from build123d import *

# Parameters (mm, degrees)
SKETCH1_W           = 39
SKETCH1_H           = 16
SKETCH1_R           = 1.5
BOSS_EXTRUDE1_DEPTH = 2
SKETCH3_W           = 25.4
SKETCH3_H           = 6.35
SKETCH3_R           = 1.5
BOSS_EXTRUDE2_DEPTH = 2.5
BOSS_EXTRUDE3_DEPTH = 6.35
SKETCH5_W           = 8
SKETCH5_H           = 15.6
BOSS_EXTRUDE4_DEPTH = 10


with BuildPart() as part:
    # Sketch1 → Boss-Extrude1 (new body)
    with BuildSketch(Plane(origin=(0, 0, 0), x_dir=(1, 0, 0), z_dir=(0, 1, 0))):
        Rectangle(SKETCH1_W, SKETCH1_H)
        with Locations(Location((-16.5, -5, 0), (0, 0, 270))):
            Circle(SKETCH1_R, mode=Mode.SUBTRACT)
        with Locations(Location((2.5, -5, 0), (0, 0, 270))):
            Circle(SKETCH1_R, mode=Mode.SUBTRACT)
    extrude(amount=BOSS_EXTRUDE1_DEPTH)

    # Sketch3 → Boss-Extrude2 (add)
    with BuildSketch(Plane(origin=(0, 2, 0), x_dir=(1, 0, 0), z_dir=(0, 1, 0))):
        with Locations((-7, -5)):
            Rectangle(SKETCH3_W, SKETCH3_H)
        with Locations(Location((-16.5, -5, 0), (0, 0, 270))):
            Circle(SKETCH3_R, mode=Mode.SUBTRACT)
        with Locations(Location((2.5, -5, 0), (0, 0, 270))):
            Circle(SKETCH3_R, mode=Mode.SUBTRACT)
    extrude(amount=BOSS_EXTRUDE2_DEPTH)

    # Sketch4 → Boss-Extrude3 (add)
    with BuildSketch(Plane.XY.offset(8.175)):
        with BuildLine():
            Line((-8.8, 13.7), (-13.5, 13.7))
            Line((-13.5, 13.7), (-13.5, 4.5))
            Line((-13.5, 4.5), (-6.999999998, 4.5))
            ThreePointArc((-6.999999998, 4.5), (-8.272792205, 5.027207793), (-8.8, 6.3))
            Line((-8.8, 6.3), (-8.8, 13.7))
        make_face()
        with BuildLine():
            ThreePointArc((-5.2, 6.3), (-5.727207793, 5.027207795), (-6.999999998, 4.5))
            Line((-6.999999998, 4.5), (-0.5, 4.5))
            Line((-0.5, 4.5), (-0.5, 13.7))
            Line((-0.5, 13.7), (-5.2, 13.7))
            Line((-5.2, 13.7), (-5.2, 6.3))
        make_face()
    extrude(amount=-BOSS_EXTRUDE3_DEPTH)

    # Sketch5 → Boss-Extrude4 (add)
    with BuildSketch(Plane(origin=(0, 2, 0), x_dir=(1, 0, 0), z_dir=(0, 1, 0))):
        with Locations((15.3, 0)):
            Rectangle(SKETCH5_W, SKETCH5_H)
    extrude(amount=BOSS_EXTRUDE4_DEPTH)


solid = part.part
Here's how the part is built. I have some questions about the finished solid (model axes, mm). A direction names the side the tool comes from. Round coordinates to 2 decimals unless told otherwise and drop trailing zeros. Write each loop counter-clockwise with the first axis right and the second up, starting at its lowest first coordinate (ties: lowest second). Pieces come first, ordered by that corner, then holes.
1. If we mould it in two halves opening along Z, with no side actions, what happens to faces 1 (the cylindrical face through (1.17, 2.22, 5.69)), 2 (the flat face through (0, 1, -8)), 3 (the flat face through (15, 12, 0)), 4 (the flat face through (-4, 7, 8.175))? For each: released by +Z, released by -Z, zero draft, split by the parting line, or undercut.
2. Suppose I cut it at B-B (x = -16.5). List the corners of the cut face in (y, z) for me (3 decimals), and give its area (3 significant figures).
3. Suppose I cut it at A-A (y = 8.25). List the corners of the cut face in (x, z) for me (3 decimals), and give its area (3 significant figures).
4. Suppose I cut it at C-C (z = 5). List the corners of the cut face in (x, y) for me.
5. Suppose I cut it at D-D (z = -4). List the corners of the cut face in (x, y) for me.
6. For faces 5 (the flat face through (-5.2, 10, 5)), 6 (the flat face through (15, 7, 7.8)), 7 (the flat face through (-4, 7, 1.825)), 8 (the flat face through (-13.5, 9, 5)), which set-ups out of +Z, -Z, +X, -X, +Y, -Y let a thin tool reach every point of the face, with its end or its side?
7. Will these pins go through, and if not, where does the flat tip stop? pin 1 Ø8 at (x, y) = (6.5, 11) entering from +Z; pin 2 Ø6 at (x, z) = (4, 0.5) entering from +Y; pin 3 Ø1.9 at (y, z) = (8, 4.5) entering from -X; pin 4 Ø8 at (x, z) = (-7, -3.5) entering from +Y.
8. I need wall thicknesses on L1, parallel to X at y = 7.5, z = 5; L2, parallel to X at y = 1.9, z = 5; L3, parallel to X at y = 2.8, z = 5. Which ranges of each line are inside material? Lowest first, please.
Answer sheet:
1. face 1: undercut
1. face 2: released by -Z
1. face 3: zero draft
1. face 4: released by +Z
2. outline: (0, -8) - (2, -8) - (2, 1.825) - (4.5, 1.825) - (4.5, 3.5) - (0, 3.5) - close; (0, 6.5) - (4.5, 6.5) - (4.5, 8.175) - (2, 8.175) - (2, 8) - (0, 8) - close
2. area: 34.4 mm2
3. outline: (-13.5, 1.825) - (-8.8, 1.825) - (-8.8, 8.175) - (-13.5, 8.175) - close; (-5.2, 1.825) - (-0.5, 1.825) - (-0.5, 8.175) - (-5.2, 8.175) - close; (11.3, -7.8) - (19.3, -7.8) - (19.3, 7.8) - (11.3, 7.8) - close
3. area: 184 mm2
4. outline: (-19.7, 2) - (-19.5, 2) - (-19.5, 0) - (-18, 0) - (-18, 4.5) - (-19.7, 4.5) - close; (-15, 0) - (1, 0) - (1, 4.5) - (-0.5, 4.5) - (-0.5, 13.7) - (-5.2, 13.7) - (-5.2, 6.3) arc R1.8 cw to (-8.8, 6.3) - (-8.8, 13.7) - (-13.5, 13.7) - (-13.5, 4.5) - (-15, 4.5) - close; (4, 0) - (19.5, 0) - (19.5, 2) - (19.3, 2) - (19.3, 12) - (11.3, 12) - (11.3, 2) - (5.7, 2) - (5.7, 4.5) - (4, 4.5) - close
5. outline: (-19.5, 0) - (19.5, 0) - (19.5, 2) - (19.3, 2) - (19.3, 12) - (11.3, 12) - (11.3, 2) - (-19.5, 2) - close
6. face 5: +Z, -Z, +Y
6. face 6: +Z, +X, +Y
6. face 7: -Z, -X, +Y
6. face 8: +Z, -Z, -X, +Y
7. pin 1: passes through
7. pin 2: stops at y = 4.5
7. pin 3: stops at x = -13.5
7. pin 4: stops at y = 2
8. L1: x = -13.5 to -8.8, -5.2 to -0.5, 11.3 to 19.3
8. L2: x = -19.5 to -18, -15 to 1, 4 to 19.5
8. L3: x = -19.7 to -18, -15 to 1, 4 to 5.7, 11.3 to 19.3
